The listing builds one solid part. Answer for the finished solid, in the listing's coordinates (mm). Coordinates: 2 decimals unless noted, no trailing zeros. Order: outer loops, then holes, each group sorted by start corner. A loop starts at its lowest first (then second) coordinate and runs counter-clockwise, first axis right, second up. Notation, with made-up numbers: (12, 59.5) -> (18, 59.5) arc R29 ccw to (18, 94.5) -> close; hole circle Ø3 at (43.25, 9). An arc over 180 degrees is marked (long way). Return JSON: item names as keys, results as strings.
from build123d import *

# Parameters (mm, degrees)
EXTRUDE_1_DEPTH          = 200
CUT_EXTRUDE_1_DEPTH      = 201.281052524
CUT_EXTRUDE_1_DEPTH_BACK = 201.281052524
SKETCH_2_R               = 2


with BuildPart() as part:
    # 草图1 → 凸台-拉伸1 (new, symmetric)
    with BuildSketch(Plane(origin=(0, 0, 0), x_dir=(0, 0, -1), z_dir=(1, 0, 0))):
        with BuildLine():
            Line((6, 7.5), (-6, 7.5))
            ThreePointArc((-6, 7.5), (-7.060660172, 7.060660172), (-7.5, 6))
            Line((-7.5, 6), (-7.5, -6))
            ThreePointArc((-7.5, -6), (-7.060660172, -7.060660172), (-6, -7.5))
            Line((-6, -7.5), (6, -7.5))
            ThreePointArc((6, -7.5), (7.060660172, -7.060660172), (7.5, -6))
            Line((7.5, -6), (7.5, 6))
            ThreePointArc((7.5, 6), (7.060660172, 7.060660172), (6, 7.5))
        make_face()
        with BuildLine():
            Line((6, 6.5), (-6, 6.5))
            ThreePointArc((-6, 6.5), (-6.353553391, 6.353553391), (-6.5, 6))
            Line((-6.5, 6), (-6.5, -6))
            ThreePointArc((-6.5, -6), (-6.353553391, -6.353553391), (-6, -6.5))
            Line((-6, -6.5), (6, -6.5))
            ThreePointArc((6, -6.5), (6.353553391, -6.353553391), (6.5, -6))
            Line((6.5, -6), (6.5, 6))
            ThreePointArc((6.5, 6), (6.353553391, 6.353553391), (6, 6.5))
        make_face(mode=Mode.SUBTRACT)
    extrude(amount=EXTRUDE_1_DEPTH, both=True)

    # 草图2 → 切除-拉伸1 (cut, two sides: drawn at the far end of the back side and taken through both)
    with BuildSketch(Plane(origin=(0, 0, 0), x_dir=(1, 0, 0), z_dir=(0, 1, 0)).offset(-CUT_EXTRUDE_1_DEPTH_BACK)):
        with Locations(Location((-180, 0, 0), (0, 0, 270))):
            Circle(SKETCH_2_R)
        with Locations(Location((-120, 0, 0), (0, 0, 270))):
            Circle(SKETCH_2_R)
        with Locations(Location((-60, 0, 0), (0, 0, 270))):
            Circle(SKETCH_2_R)
        with Locations(Location((0, 0, 0), (0, 0, 270))):
            Circle(SKETCH_2_R)
        with Locations(Location((60, 0, 0), (0, 0, 270))):
            Circle(SKETCH_2_R)
        with Locations(Location((120, 0, 0), (0, 0, 270))):
            Circle(SKETCH_2_R)
        with Locations(Location((180, 0, 0), (0, 0, 270))):
            Circle(SKETCH_2_R)
    extrude(amount=CUT_EXTRUDE_1_DEPTH + CUT_EXTRUDE_1_DEPTH_BACK, mode=Mode.SUBTRACT)


solid = part.part
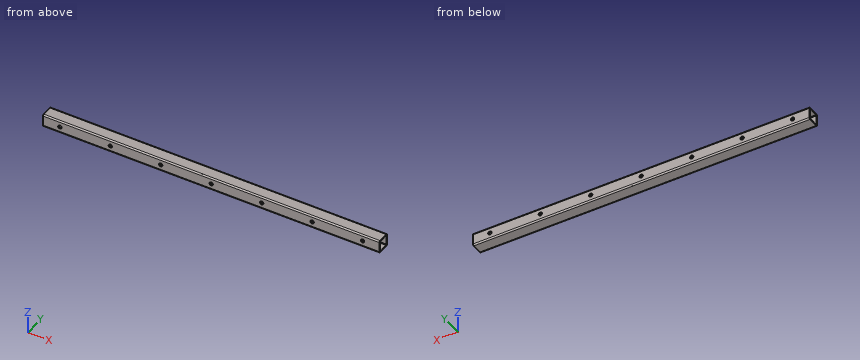
1. Consider line 1 (Y direction, x = -127.5, z = 3.75); line 2 (Y direction, x = 47, z = 6.25). Determine where each line is inside the solid, lowest interval first. Write a range as from..to.
Answer block:
{"line 1": "y = -7.5..-6.5, 6.5..7.5", "line 2": "y = -7.48..-6.43, 6.43..7.48"}
2. The part is cut by section B-B on x = -104. Give the vertices of the cut face in (y, z).
Answer block:
{"outline": "(-7.5, -6) arc R1.5 ccw to (-6, -7.5) -> (6, -7.5) arc R1.5 ccw to (7.5, -6) -> (7.5, 6) arc R1.5 ccw to (6, 7.5) -> (-6, 7.5) arc R1.5 ccw to (-7.5, 6) -> close; hole (-6.5, -6) arc R0.5 ccw to (-6, -6.5) -> (6, -6.5) arc R0.5 ccw to (6.5, -6) -> (6.5, 6) arc R0.5 ccw to (6, 6.5) -> (-6, 6.5) arc R0.5 ccw to (-6.5, 6) -> close"}
3. This flat-tipped pin is pushed along its axis until it touches: pin 1 Ø2.5 at (x, z) = (-180, 0) entering from -Y. Where does it stop, or does it pass through?
Answer block:
{"pin 1": "passes through"}
4. The part is cut by section A-A on y = 1.5. Give the vertices of the cut face in (x, z), and give its area (3 significant figures).
Answer block:
{"outline": "(-200, -7.5) -> (200, -7.5) -> (200, -6.5) -> (-200, -6.5) -> close; (-200, 6.5) -> (200, 6.5) -> (200, 7.5) -> (-200, 7.5) -> close", "area": "800 mm2"}
